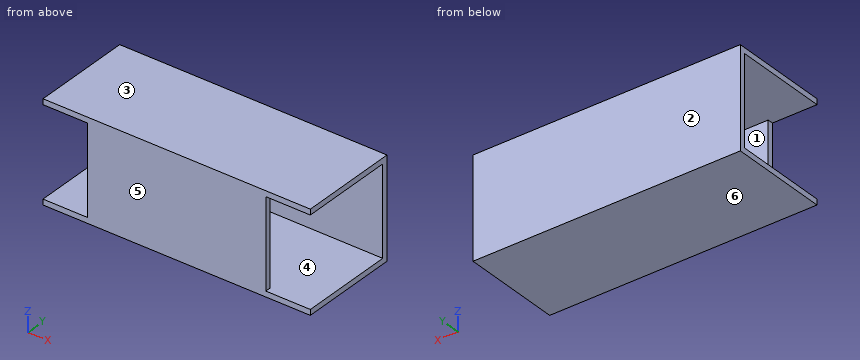
from build123d import *

# Parameters (mm, degrees)
F0_W     = 203.2
F0_H     = 114.3
F1_DEPTH = 114.3
F2_W     = 101.6
F2_H     = 101.6
F3_DEPTH = 203.201
F4_W     = 107.95
F4_H     = 6.35
F5_DEPTH = 50.8
F6_W     = 107.95
F6_H     = 6.35
F7_DEPTH = 50.8


with BuildPart() as f1:
    # F0 (on Top) → F1 (new body)
    with BuildSketch(Plane.XY):
        Rectangle(F0_W, F0_H)
    extrude(amount=F1_DEPTH)

    # F2 (on face) → F3 (cut, through all)
    with BuildSketch(Plane(origin=(-101.6, 0, 0), x_dir=(0, -1, 0), z_dir=(-1, 0, 0))):
        with Locations((0, 57.15)):
            Rectangle(F2_W, F2_H)
    extrude(amount=-F3_DEPTH, mode=Mode.SUBTRACT)

    # F4 (on face) → F5 (join)
    with BuildSketch(Plane.YZ.offset(101.6)):
        Polygon((57.15, 0), (57.15, 114.3), (50.8, 114.3), (50.8, 107.95), (50.8, 6.35), (50.8, 0), align=None)
        with Locations((-3.175, 111.125)):
            Rectangle(F4_W, F4_H)
        with Locations((-3.175, 3.175)):
            Rectangle(F4_W, F4_H)
    extrude(amount=F5_DEPTH)

    # F6 (on face) → F7 (join)
    with BuildSketch(Plane(origin=(-101.6, 0, 0), x_dir=(0, -1, 0), z_dir=(-1, 0, 0))):
        Polygon((-50.8, 114.3), (-57.15, 114.3), (-57.15, 0), (-50.8, 0), (-50.8, 6.35), (-50.8, 107.95), align=None)
        with Locations((3.175, 111.125)):
            Rectangle(F6_W, F6_H)
        with Locations((3.175, 3.175)):
            Rectangle(F6_W, F6_H)
    extrude(amount=F7_DEPTH)


solid = f1.part
CAD build for the part. Positions are in the model's coordinates, mm. Face numbers are marked on the shaded views. A direction names the side the tool comes from. Round coordinates to 2 decimals unless told otherwise and drop trailing zeros. Loops run counter-clockwise (first coordinate to the right, second up) from the corner with the lowest first, then second, coordinate; pieces in that order, holes last.
(1) Cut at C-C (x = 51). Give the cut face in (y, z), plus the area to 3 significant figures.
(2) Two-plate mould, pull along Z, no slides. Class the marked faces 3, 4, 5 and 6: +Z half, -Z half, draft (parallel to the pull), parting line (faces both ways), or undercut.
(3) Which spindle directions (+Z, -Z, +X, -X, +Y, -Y) get a long thin tool onto all of the face, cutting with end or side? Do the marked faces 1 and 2. Say none if no direction does.
(4) Drop flat-ended pins along their axis: pin 1 (1.9 mm diameter, centred on y = -54, z = 57.5, fed in from -X); pin 2 (3 mm diameter, centred on y = -52.5, z = 66.5, fed in from +X). Give the stop position or say it passes through.
(5) Wall check: line 1 along Z through (x, y) = (7.5, 30); line 2 along Y through (x, z) = (-85, 13); line 3 along Y through (x, z) = (125, 48). Give the ranges that are in metal, low to high.
(6) Cut at D-D (x = 127.5). Give the cut face in (y, z).
(7) Cut at A-A (y = 36). Give the cut face in (x, z), plus the area to 3 significant figures.
(8) Cut at B-B (z = 95). Give the cut face in (x, y).
Findings below:
1. outline: (-57.15, 0) - (57.15, 0) - (57.15, 114.3) - (-57.15, 114.3) - close; hole (-50.8, 6.35) - (50.8, 6.35) - (50.8, 107.95) - (-50.8, 107.95) - close
1. area: 2,740 mm2
2. face 3: +Z half
2. face 4: undercut
2. face 5: draft
2. face 6: -Z half
3. face 1: +X, -X
3. face 2: +Z, -Z, +X, -X, +Y
4. pin 1: stops at x = -101.6
4. pin 2: stops at x = 101.6
5. line 1: z = 0 to 6.35, 107.95 to 114.3
5. line 2: y = -57.15 to -50.8, 50.8 to 57.15
5. line 3: y = 50.8 to 57.15
6. outline: (-57.15, 0) - (57.15, 0) - (57.15, 114.3) - (-57.15, 114.3) - (-57.15, 107.95) - (50.8, 107.95) - (50.8, 6.35) - (-57.15, 6.35) - close
7. outline: (-152.4, 0) - (152.4, 0) - (152.4, 6.35) - (-152.4, 6.35) - close; (-152.4, 107.95) - (152.4, 107.95) - (152.4, 114.3) - (-152.4, 114.3) - close
7. area: 3,870 mm2
8. outline: (-152.4, 50.8) - (152.4, 50.8) - (152.4, 57.15) - (-152.4, 57.15) - close; (-101.6, -57.15) - (101.6, -57.15) - (101.6, -50.8) - (-101.6, -50.8) - close
